```python
from build123d import *

# Parameters (mm, degrees)
BOSS_EXTRUDE1_START     = -3
SKETCH1_W               = 20
SKETCH1_H               = 6
BOSS_EXTRUDE1_DEPTH     = 6
BOSS_EXTRUDE2_REACH     = 713.032
SKETCH2_W               = 40
SKETCH2_H               = 6
SKETCH3_R               = 1.5
CUT_EXTRUDE1_DEPTH      = 730.905928511
FILLET1_R               = 1
CUT_EXTRUDE3_DEPTH      = 730.725112263
CUT_EXTRUDE3_DEPTH_BACK = 730.725112263
SKETCH5_R               = 1.5
CUT_EXTRUDE4_DEPTH      = 730.725112263


with BuildPart() as part:
    # Sketch1 → Boss-Extrude1 (new body)
    with BuildSketch(Plane.XY.offset(BOSS_EXTRUDE1_START)):
        with Locations((701, 123)):
            Rectangle(SKETCH1_W, SKETCH1_H)
    extrude(amount=BOSS_EXTRUDE1_DEPTH)

    # Boss-Extrude2: up to this plane
    boss_extrude2_end = Plane(origin=(261.902222158, 420.028150272, 347.5), z_dir=(-0.5291046610932348, -0.8485565730164449, 0))
    # Sketch2 → Boss-Extrude2 (add, up to the surface)
    with BuildSketch(Plane(origin=(0, 126, 0), x_dir=(1, 0, 0), z_dir=(0, 1, 0)), mode=Mode.PRIVATE) as boss_extrude2_sk1:
        with Locations((691, 0)):
            Rectangle(SKETCH2_W, SKETCH2_H)
    boss_extrude2_tool1 = split(extrude(boss_extrude2_sk1.sketch, amount=BOSS_EXTRUDE2_REACH, mode=Mode.PRIVATE), bisect_by=boss_extrude2_end, keep=Keep.BOTH, mode=Mode.PRIVATE)
    add(boss_extrude2_tool1.solids().sort_by_distance((691, 126, 0))[0])

    # Sketch3 → Cut-Extrude1 (cut, through all)
    with BuildSketch(Plane.XY.offset(3)):
        with Locations((691, 126)):
            Circle(SKETCH3_R)
    extrude(amount=-CUT_EXTRUDE1_DEPTH, mode=Mode.SUBTRACT)

    # Fillet1
    fillet1_edges = [part.edges().sort_by_distance(p)[0] for p in [
        (671, 164.941397093, 0),
    ]]
    fillet(fillet1_edges, radius=FILLET1_R)

    # Sketch4 → Cut-Extrude3 (cut, two sides)
    with BuildSketch(Plane.XY.offset(3)) as cut_extrude3_sk:
        Polygon((688.717930776, 153.893648414), (685.54330281, 148.802308976), (711, 132.929169143), (714.174627967, 138.020508582), align=None)
    extrude(amount=CUT_EXTRUDE3_DEPTH, mode=Mode.SUBTRACT)
    extrude(cut_extrude3_sk.sketch, amount=-CUT_EXTRUDE3_DEPTH_BACK, mode=Mode.SUBTRACT)

    # Sketch5 → Cut-Extrude4 (cut, through all)
    with BuildSketch(Plane.XY.offset(3)):
        with Locations((685.54330281, 148.802308976)):
            Circle(SKETCH5_R)
    extrude(amount=-CUT_EXTRUDE4_DEPTH, mode=Mode.SUBTRACT)


solid = part.part
```
Verification items for the finished model (mm, model axes). A direction names the side the tool comes from. Coordinates: 2 decimals unless noted, no trailing zeros. Write each loop counter-clockwise with the first axis right and the second up, starting at its lowest first coordinate (ties: lowest second). Pieces come first, ordered by that corner, then holes. Notation, with made-up numbers: (27, 1.5) - (65, 1.5) arc R14 cw to (65, 9.5) - close; hole circle Ø11 at (27, 70.5). An arc over 180 degrees is marked (long way). One line per question, with ' | ' between items. Start each with the question number.
1. Material ranges on line 1 along Y through (x, z) = (686.5, 0.5); line 2 along X through (y, z) = (122.5, -1); line 3 along Y through (x, z) = (675, 2), recorded low to high.
2. Draft check along Y on faces 1 (the flat face through (686, 137, -3)), 2 (the flat face through (701, 120, 0)), 3 (the cylindrical face through (692.095, 127.025, 0.042)). Enter one of: released by +Y, released by -Y, zero draft, split by the parting line, or undercut.
3. Section check C-C (y = 161.5). Enter the section's corners in (x, z).
4. Access from +Z, -Z, +X, -X, +Y, -Y to the whole of each face (thin tool, end or side, straight path). Record for faces 4 (the flat face through (680, 126, 0)), 5 (the flat face through (687.544, 152.011, 0.042)), 6 (the cylindrical face through (671.502, 164.006, 0.042)).
5. Section check A-A (z = 1.75). Enter the section's corners in (x, y), plus the area to 3 significant figures.
6. Gauge pin test, flat ends, axial feed: P1, Ø1, axis at x = 701, z = -2.5, coming from the +Y side; P2, Ø4, axis at x = 691, y = 126, coming from the +Z side; P3, Ø3, axis at y = 153, z = -1, coming from the +X side; P4, Ø1.3, axis at y = 123.5, z = -0.5, coming from the -X side. Record the tip position at first contact, or that the pin passes through.
7. Section check B-B (x = 696). Enter the section's corners in (y, z), plus the area to 3 significant figures.
Computed values:
1) line 1: 126 to 147.65, 150.34 to 155.28 | line 2: 691 to 711 | line 3: 126 to 162.45
2) face 1: zero draft | face 2: released by -Y | face 3: undercut
3) outline: (671, -3) - (676.52, -3) - (676.52, 3) - (671, 3) - close
4) face 4: +Z, -Z, -X, -Y | face 5: +Z, -Z, +X | face 6: +Z, -Z, +Y
5) outline: (671, 126) - (689.5, 126) arc R1.5 cw (long way) to (691, 124.5) - (691, 120) - (711, 120) - (711, 132.93) - (686.82, 148.01) arc R1.5 cw (long way) to (686.34, 150.08) - (688.72, 153.89) - (672.53, 163.99) arc R1 ccw to (671, 163.14) - close | area: 999 mm²
6) P1: y = 139.48 | P2: z = 3 | P3: x = 688.72 | P4: x = 691
7) outline: (120, -3) - (142.28, -3) - (142.28, 3) - (120, 3) - close | area: 134 mm²
